Geometry check sheet. Reference: the model listing, model coordinates, mm. A direction names the side the tool comes from. Round coordinates to 2 decimals unless told otherwise and drop trailing zeros. Order: outer loops, then holes, each group sorted by start corner. A loop starts at its lowest first (then second) coordinate and runs counter-clockwise, first axis right, second up. Notation, with made-up numbers: (-22.5, 4.5) - (6.5, 4.5) arc R17 cw to (6.5, 22.5) - close; hole circle Ø5 at (-25.5, -30.5). An arc over 180 degrees is marked (long way). One line per question, with ' | ' between items. Start each with the question number.
Q1. Sectioned sample at C-C, the plane x = 21.5. Enter the section's corners in (y, z), then the cut area to 3 significant figures.
Q2. Gauge pin test, flat ends, axial feed: P1, Ø2.5, axis at y = 4, z = -39, coming from the -X side; P2, Ø3, axis at x = -32.5, y = -2, coming from the +Z side; P3, Ø1, axis at y = 5.5, z = 23, coming from the +X side. Record the tip position at first contact, or that the pin passes through.
Q3. Sectioned sample at D-D, the plane z = -21.5. Enter the section's corners in (x, y), then the cut area to 3 significant figures.
Q4. Tool access check on faces 4 (the face through (-12.8, 12, 38)), 5 (the face through (-2, 18, -26)), 6 (the face through (-20, 8, -38)), 7 (the face through (8.4, 12.07, 40.26)), 8 (the face through (-0.2, 17, 4.3)). Record the directions out of +Z, -Z, +X, -X, +Y, -Y that give a thin tool (end or side, any length) a straight path to the whole face; none if there is none.
Q5. Sectioned sample at A-A, the plane z = 0. Enter the section's corners in (x, y).
Q6. Material ranges on line 1 along Y through (x, z) = (-10, 39.9); line 2 along Z through (x, y) = (35, 5); line 3 along Z through (x, y) = (-11, 10.5), recorded low to high.
Q7. Sectioned sample at B-B, the plane y = 3. Enter the section's corners in (x, z), then the cut area to 3 significant figures.
Q8. Mould release check, pull along X, two halves, no side actions. Record for faces 1 (the face through (0, 8, 41)), 2 (the face through (-20, 8, 38)), 3 (the face through (-11.6, 12.07, -39.99)): +X half, -X half, draft (parallel to the pull), parting line (faces both ways), or undercut.
```python
from build123d import *

# Parameters (mm, degrees)
SKETCH_1_R           = 41
SKETCH_1_R_2         = 39
EXTRUDE_1_DEPTH      = 20
EXTRUDE_START        = -14
EXTRUDE_2_DEPTH      = 14
EXTRUDE_START_2      = -3
SKETCH_3_R           = 4
SKETCH_3_R_2         = 1.6
EXTRUDE_3_DEPTH      = 3
CUT_EXTRUDE_3_DEPTH  = 3
EXTRUDE_5_DEPTH      = 10
EXTRUDE_5_DEPTH_BACK = 15
SKETCH_1_2_R         = 41
SKETCH_1_2_R_2       = 39
EXTRUDE_START_3      = 10
EXTRUDE_7_DEPTH      = 10
EXTRUDE_8_DEPTH      = 10
EXTRUDE_8_DEPTH_BACK = 5
CUT_EXTRUDE_4_DEPTH  = 80
EXTRUDE_START_4      = -24
EXTRUDE_10_DEPTH     = 24
EXTRUDE_9_DEPTH      = 10
EXTRUDE_9_DEPTH_BACK = 1.5
CUT_EXTRUDE_6_DEPTH  = 10
SKETCH_16_R          = 1.6
CUT_EXTRUDE_7_DEPTH  = 103
SKETCH_18_R          = 1.6
CUT_EXTRUDE_8_DEPTH  = 10
SKETCH_18_4_R        = 1.6
CUT_EXTRUDE_9_DEPTH  = 10


# Read off the part's stored shape, not the designer's step: the extrude step
with BuildPart() as part:
    # Sketch 1 → Extrude 1 (new body)
    with BuildSketch(Plane(origin=(0, 0, 0), x_dir=(1, 0, 0), z_dir=(0, 1, 0))):
        with Locations(Location((0, 0, 0), (0, 0, 270))):
            Circle(SKETCH_1_R)
        with Locations(Location((0, 0, 0), (0, 0, 270))):
            Circle(SKETCH_1_R_2, mode=Mode.SUBTRACT)
    extrude(amount=EXTRUDE_1_DEPTH)

    # Sketch 2 → Extrude 2 (add)
    with BuildSketch(Plane(origin=(0, 20, 0), x_dir=(1, 0, 0), z_dir=(0, 1, 0)).offset(EXTRUDE_START)):
        with BuildLine():
            Line((-20, -41), (3.5e-08, -41))
            ThreePointArc((3.5e-08, -41), (-10.333598732, -39.676400256), (-20, -35.791060336))
            Line((-20, -35.791060336), (-20, -41))
        make_face()
        with BuildLine():
            Line((3.5e-08, -41), (20, -41))
            Line((20, -41), (20, -35.791060336))
            ThreePointArc((20, -35.791060336), (10.333598766, -39.676400247), (3.5e-08, -41))
        make_face()
    extrude(amount=EXTRUDE_2_DEPTH)

    # Sketch 3 → Extrude 3 (add)
    with BuildSketch(Plane(origin=(0, 20, 0), x_dir=(1, 0, 0), z_dir=(0, 1, 0)).offset(EXTRUDE_START_2)):
        with BuildLine():
            Line((-2, 38.948684188), (-2, 13.351029923))
            ThreePointArc((-2, 13.351029923), (-11.691342951, 6.75), (-12.56233108, -4.943464154))
            Line((-12.56233108, -4.943464154), (-34.730549951, -17.742291287))
            ThreePointArc((-34.730549951, -17.742291287), (-33.774990748, -19.5), (-32.730549951, -21.206392902))
            Line((-32.730549951, -21.206392902), (-10.56233108, -8.407565769))
            ThreePointArc((-10.56233108, -8.407565769), (0, -13.5), (10.56233108, -8.407565769))
            Line((10.56233108, -8.407565769), (32.730549951, -21.206392902))
            ThreePointArc((32.730549951, -21.206392902), (33.774990748, -19.5), (34.730549951, -17.742291287))
            Line((34.730549951, -17.742291287), (12.56233108, -4.943464154))
            ThreePointArc((12.56233108, -4.943464154), (11.691342951, 6.75), (2, 13.351029923))
            Line((2, 13.351029923), (2, 38.948684188))
            ThreePointArc((2, 38.948684188), (0, 39), (-2, 38.948684188))
        make_face()
        with Locations(Location((0, 0, 0), (0, 0, 270))):
            Circle(SKETCH_3_R, mode=Mode.SUBTRACT)
        with Locations(Location((-8, 0, 0), (0, 0, 270))):
            Circle(SKETCH_3_R_2, mode=Mode.SUBTRACT)
        with Locations(Location((8, 0, 0), (0, 0, 270))):
            Circle(SKETCH_3_R_2, mode=Mode.SUBTRACT)
    extrude(amount=EXTRUDE_3_DEPTH)

    # Sketch 7 → Cut-Extrude 3 (cut)
    with BuildSketch(Plane.XZ.offset(-6)):
        with BuildLine():
            Line((0, 41), (-20, 41))
            Line((-20, 41), (-20, 35.791060336))
            ThreePointArc((-20, 35.791060336), (-10.333598749, 39.676400251), (0, 41))
        make_face()
        with BuildLine():
            Line((20, 41), (0, 41))
            ThreePointArc((0, 41), (10.333598749, 39.676400251), (20, 35.791060336))
            Line((20, 35.791060336), (20, 41))
        make_face()
    extrude(amount=-CUT_EXTRUDE_3_DEPTH, mode=Mode.SUBTRACT)

    # Sketch 1_2 → Extrude 5 (add, two sides: drawn at the far end of the back side and taken through both)
    with BuildSketch(Plane(origin=(0, 0, 0), x_dir=(1, 0, 0), z_dir=(0, 1, 0)).offset(-EXTRUDE_5_DEPTH_BACK)):
        with Locations(Location((0, 0, 0), (0, 0, 270))):
            Circle(SKETCH_1_2_R)
        with Locations(Location((0, 0, 0), (0, 0, 92.939534486))):
            Circle(SKETCH_1_2_R_2, mode=Mode.SUBTRACT)
    extrude(amount=EXTRUDE_5_DEPTH + EXTRUDE_5_DEPTH_BACK)

    # Sketch 7_4 → Extrude 7 (add)
    with BuildSketch(Plane.XZ.offset(-6).offset(EXTRUDE_START_3)):
        with BuildLine():
            Line((0, 41), (-20, 41))
            Line((-20, 41), (-20, 35.791060336))
            ThreePointArc((-20, 35.791060336), (-10.333598749, 39.676400251), (0, 41))
        make_face()
        with BuildLine():
            Line((20, 41), (0, 41))
            ThreePointArc((0, 41), (10.333598749, 39.676400251), (20, 35.791060336))
            Line((20, 35.791060336), (20, 41))
        make_face()
    extrude(amount=-EXTRUDE_7_DEPTH)

    # Sketch 7_5 → Extrude 8 (add, two sides: drawn at the far end of the back side and taken through both)
    with BuildSketch(Plane.XZ.offset(-6).offset(-EXTRUDE_8_DEPTH_BACK)):
        with BuildLine():
            Line((0, 41), (-20, 41))
            Line((-20, 41), (-20, 35.791060336))
            ThreePointArc((-20, 35.791060336), (-10.333598749, 39.676400251), (0, 41))
        make_face()
        with BuildLine():
            Line((20, 41), (0, 41))
            ThreePointArc((0, 41), (10.333598749, 39.676400251), (20, 35.791060336))
            Line((20, 35.791060336), (20, 41))
        make_face()
    extrude(amount=EXTRUDE_8_DEPTH + EXTRUDE_8_DEPTH_BACK)

    # Sketch 4 → Cut-Extrude 4 (cut)
    with BuildSketch(Plane.XY.offset(41)):
        Polygon((-10, 8.766838493), (-7.2, 10.383419246), (-7.2, 13.616580754), (-10, 15.233161507), (-12.8, 13.616580754), (-12.8, 10.383419246), align=None)
        Polygon((12.8, 10.383419246), (10, 8.766838493), (7.2, 10.383419246), (7.2, 13.616580754), (10, 15.233161507), (12.8, 13.616580754), align=None)
    extrude(amount=-CUT_EXTRUDE_4_DEPTH, mode=Mode.SUBTRACT)

    # Extrude 10 outline → Extrude 10 (add)
    with BuildSketch(Plane(origin=(0, 20, 0), x_dir=(1, 0, 0), z_dir=(0, 1, 0)).offset(EXTRUDE_START_4)):
        with BuildLine():
            Line((20, 35.791060336), (20, 41))
            Line((20, 41), (8e-08, 41))
            ThreePointArc((8e-08, 41), (6.403124277, 40.496913456), (12.649110641, 39))
            ThreePointArc((12.649110641, 39), (12.72457916, 38.975442079), (12.8, 38.950738119))
            ThreePointArc((12.8, 38.950738119), (16.475918515, 37.543895763), (20, 35.791060336))
        make_face()
        with BuildLine():
            ThreePointArc((-12.649110641, 39), (-6.403124198, 40.496913469), (8e-08, 41))
            Line((8e-08, 41), (-20, 41))
            Line((-20, 41), (-20, 35.791060336))
            ThreePointArc((-20, 35.791060336), (-16.475918515, 37.543895763), (-12.8, 38.950738119))
            ThreePointArc((-12.8, 38.950738119), (-12.72457916, 38.975442079), (-12.649110641, 39))
        make_face()
    extrude(amount=EXTRUDE_10_DEPTH)

    # Sketch 4_3 → Extrude 9 (add, two sides: drawn at the far end of the back side and taken through both)
    with BuildSketch(Plane.XY.offset(41).offset(-EXTRUDE_9_DEPTH_BACK)):
        Polygon((-10, 8.766838493), (-7.2, 10.383419246), (-7.2, 13.616580754), (-10, 15.233161507), (-12.8, 13.616580754), (-12.8, 10.383419246), align=None)
        Polygon((12.8, 10.383419246), (10, 8.766838493), (7.2, 10.383419246), (7.2, 13.616580754), (10, 15.233161507), (12.8, 13.616580754), align=None)
    extrude(amount=EXTRUDE_9_DEPTH + EXTRUDE_9_DEPTH_BACK)

    # Sketch 13 → Cut-Extrude 6 (cut)
    with BuildSketch(Plane.XY.offset(51)):
        Polygon((10, 15.233161507), (7.2, 13.616580754), (7.2, 10.383419246), (10, 8.766838493), (12.8, 10.383419246), (12.8, 13.616580754), align=None)
        Polygon((-10, 15.233161507), (-12.8, 13.616580754), (-12.8, 10.383419246), (-10, 8.766838493), (-7.2, 10.383419246), (-7.2, 13.616580754), align=None)
    extrude(amount=-CUT_EXTRUDE_6_DEPTH, mode=Mode.SUBTRACT)

    # Sketch 16 → Cut-Extrude 7 (cut)
    with BuildSketch(Plane.XY.offset(41)):
        with Locations((-10, 12)):
            Circle(SKETCH_16_R)
        with Locations((10, 12)):
            Circle(SKETCH_16_R)
    extrude(amount=-CUT_EXTRUDE_7_DEPTH, mode=Mode.SUBTRACT)

    # Sketch 18 → Cut-Extrude 8 (cut)
    with BuildSketch(Plane(origin=(0, 20, 0), x_dir=(1, 0, 0), z_dir=(0, 1, 0))):
        with Locations(Location((0, 9.5, 0), (0, 0, 270))):
            Circle(SKETCH_18_R)
    extrude(amount=-CUT_EXTRUDE_8_DEPTH, mode=Mode.SUBTRACT)

    # Sketch 18_4 → Cut-Extrude 9 (cut)
    with BuildSketch(Plane(origin=(0, 20, 0), x_dir=(1, 0, 0), z_dir=(0, 1, 0))):
        with Locations(Location((0, 9.5, 0), (0, 0, 270))):
            Circle(SKETCH_18_4_R)
        with Locations(Location((0, -9.5, 0), (0, 0, 270))):
            Circle(SKETCH_18_4_R)
    extrude(amount=-CUT_EXTRUDE_9_DEPTH, mode=Mode.SUBTRACT)


solid = part.part
```
Determined:
1) outline: (-15, -34.91) - (20, -34.91) - (20, -32.54) - (-15, -32.54) - close; (-15, 32.54) - (20, 32.54) - (20, 34.91) - (-15, 34.91) - close; (17, 10.1) - (20, 10.1) - (20, 14.72) - (17, 14.72) - close | area: 180 mm2
2) P1: stops at x = -20 | P2: stops at z = 26.83 | P3: stops at x = 34.27
3) outline: (-34.91, -15) - (-32.54, -15) - (-32.54, 20) - (-34.91, 20) - close; (-2, 17) - (2, 17) - (2, 20) - (-2, 20) - close; (32.54, -15) - (34.91, -15) - (34.91, 20) - (32.54, 20) - close | area: 178 mm2
4) face 4: none | face 5: +Y, -Y | face 6: -Z, -X, +Y, -Y | face 7: +Z, -Z | face 8: -Y
5) outline: (-41, -15) - (-39, -15) - (-39, 20) - (-41, 20) - close; (-13.5, 17) - (-9.6, 17) - (-9.6, 20) - (-13.5, 20) - close; (-6.4, 17) - (-4, 17) - (-4, 20) - (-6.4, 20) - close; (4, 17) - (6.4, 17) - (6.4, 20) - (4, 20) - close; (9.6, 17) - (13.5, 17) - (13.5, 20) - (9.6, 20) - close; (39, -15) - (41, -15) - (41, 20) - (39, 20) - close
6) line 1: y = -4 to 10.4, 13.6 to 20 | line 2: z = -21.35 to -17.2, 17.2 to 21.35 | line 3: z = -41 to -39, 39.5 to 41
7) outline: (-20, -41) - (20, -41) - (20, -35.79) arc R41 ccw to (20, 35.79) - (20, 41) - (-20, 41) - (-20, 35.79) arc R41 ccw to (-20, -35.79) - close; hole circle Ø78 at (0, 0) | area: 638 mm2
8) face 1: draft | face 2: -X half | face 3: undercut
